Input: part model. Units: mm. Frame: model coordinates. Coordinates: 2 decimals unless noted, no trailing zeros. Order: outer loops, then holes, each group sorted by start corner. A loop starts at its lowest first (then second) coordinate and runs counter-clockwise, first axis right, second up. Notation, with made-up numbers: (30, 38) - (56, 38) arc R26 ccw to (56, 59) - close; hole circle Ø4 at (66, 37). An arc over 180 degrees is marked (long way). One line per question, with ' | ' between items. Start each with the question number.
Autodesk Inventor part; units mm, degrees
ref_plane "YZ Plane" through (0, 0, 0) normal (1, 0, 0) x (0, 1, 0)
ref_plane "XZ Plane" through (0, 0, 0) normal (0, 1, 0) x (-1, 0, 0)
ref_plane "XY Plane" through (0, 0, 0) normal (0, 0, 1) x (1, 0, 0)
sketch "Skizze1" plane through (0, 0, 0) normal (1, 0, 0) x (0, 1, 0)
  line L0 (20, 20) -> (-20, 20)
  line L1 (-20, 20) -> (-20, -20)
  line L2 (-20, -20) -> (20, -20)
  line L3 (20, -20) -> (20, 20)
  point P0 (0, 0)
  dimension "d0" = 40
  dimension "d1" = 40
  dimension "d2" = 20
  dimension "d3" = 20
extrude "Extrusion1" add sketch "Skizze1" along normal blind 10
sketch "Skizze2" plane through (10, 0, 0) normal (1, 0, 0) x (0, 0, -1)
  circle A0 centre (-15, 15) radius 3
  circle A1 centre (-15, -15) radius 3
  circle A2 centre (15, -15) radius 3
  circle A3 centre (15, 15) radius 3
  point P0 (0, 0)
  point P1 (0, 0)
  dimension "d7" = 6
  dimension "d8" = 15
  dimension "d9" = 15
  dimension "d14" = 360
extrude "Extrusion2" cut sketch "Skizze2" against normal through all
sketch "Skizze3" plane through (10, 0, 0) normal (1, 0, 0) x (0, 0, -1)
  circle A0 centre (-9.1, 0) radius 1.4
  line L0 (0, 22.3983) -> (0, -21.9034) construction
  circle A1 centre (9.1, 0) radius 1.4
  point P0 (0, 0)
  dimension "d16" = 2.8
  dimension "d17" = 9.1
extrude "Extrusion3" cut sketch "Skizze3" against normal through all
properties part number "AdapterplatteGong_2025-03-27v00r00grm"
(1) Pin query (flat end, axial travel): pin 1 (3.5 mm diameter, centred on y = 15, z = -15, fed in from +X). Return the tip coordinate at first contact, or that it passes through.
(2) Section D-D (x = 2.25). Output: boundary loops of the cut face in (y, z), then the cut area to 3 significant figures.
(3) Section C-C (z = -15). Output: boundary loops of the cut face in (x, y).
(4) Draft query along Y for faces 1 (the face through (5, 0, 20)), 2 (the face through (5, -20, 0)), 3 (the face through (5.07, 0.06, 10.5)). Return one class per face: +Y half, -Y half, draft (parallel to the pull), parting line (faces both ways), or undercut.
(5) Material intervals for line 1 along Y through (x, z) = (5.5, -15); line 2 along Z through (x, y) = (2.5, -14.5); line 3 along Z through (x, y) = (7, 1), sorted ascending. Write a range as from..to.
(6) Section B-B (y = 0). Output: boundary loops of the cut face in (x, z), then the cut area to 3 significant figures.
(7) Section A-A (z = -9.1). Output: boundary loops of the cut face in (x, y), then the cut area to 3 significant figures.
Worked answers:
1) pin 1: passes through
2) outline: (-20, -20) - (20, -20) - (20, 20) - (-20, 20) - close; hole circle Ø6 at (-15, -15); hole circle Ø6 at (-15, 15); hole circle Ø2.8 at (0, -9.1); hole circle Ø2.8 at (0, 9.1); hole circle Ø6 at (15, -15); hole circle Ø6 at (15, 15) | area: 1,470 mm²
3) outline: (0, -20) - (10, -20) - (10, -18) - (0, -18) - close; (0, -12) - (10, -12) - (10, 12) - (0, 12) - close; (0, 18) - (10, 18) - (10, 20) - (0, 20) - close
4) face 1: draft | face 2: -Y half | face 3: undercut
5) line 1: y = -20..-18, -12..12, 18..20 | line 2: z = -20..-17.96, -12.04..12.04, 17.96..20 | line 3: z = -20..-10.08, -8.12..8.12, 10.08..20
6) outline: (0, -20) - (10, -20) - (10, -10.5) - (0, -10.5) - close; (0, -7.7) - (10, -7.7) - (10, 7.7) - (0, 7.7) - close; (0, 10.5) - (10, 10.5) - (10, 20) - (0, 20) - close | area: 344 mm²
7) outline: (0, -20) - (10, -20) - (10, -1.4) - (0, -1.4) - close; (0, 1.4) - (10, 1.4) - (10, 20) - (0, 20) - close | area: 372 mm²
